Autodesk Inventor part; units mm, degrees
ref_plane "YZ Plane" through (0, 0, 0) normal (1, 0, 0) x (0, 1, 0)
ref_plane "XZ Plane" through (0, 0, 0) normal (0, 1, 0) x (-1, 0, 0)
ref_plane "XY Plane" through (0, 0, 0) normal (0, 0, 1) x (1, 0, 0)
sketch "Sketch1" plane through (0, 0, 0) normal (0, 0, 1) x (1, 0, 0)
  circle A0 centre (0, 0) radius 17.5
  dimension "d0" = 35
extrude "Extrusion1" add sketch "Sketch1" along normal blind 4.5
sketch "Sketch2" plane through (0, 0, 4.5) normal (0, 0, 1) x (1, 0, 0)
  circle A0 centre (0, 0) radius 17.5
  circle A1 centre (0, 0) radius 11
  dimension "d3" = 22
extrude "Extrusion2" add sketch "Sketch2" along normal blind 6.5 contours A1
sketch "Sketch3" plane through (0, 0, 11) normal (0, 0, 1) x (1, 0, 0)
  circle A0 centre (0, 0) radius 11
  circle A1 centre (0, 0) radius 6
  dimension "d6" = 12
extrude "Extrusion3" cut sketch "Sketch3" against normal through all contours A1
properties part number "culinder cap"
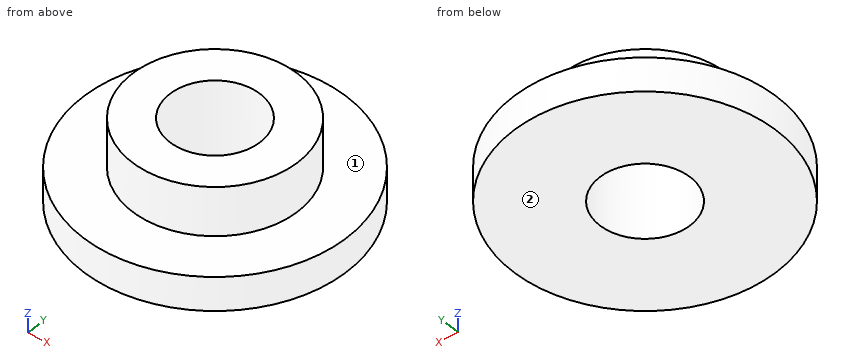
Geometry: final body of the model. Coordinates: model frame, mm. Face numbers are marked on the shaded views. A direction names the side the tool comes from. Round coordinates to 2 decimals unless told otherwise and drop trailing zeros. Loops run counter-clockwise (first coordinate to the right, second up) from the corner with the lowest first, then second, coordinate; pieces in that order, holes last. Notation, with made-up numbers: (-13.5, 14) -> (-8.5, 14) arc R22 ccw to (-8.5, 49) -> close; hole circle Ø10 at (78, 6). An arc over 180 degrees is marked (long way). Write each question's results on one line, items separated by ' | '.
Item 1: Pin query (flat end, axial travel): pin 1 Ø4 at (y, z) = (3.5, 6) entering from +X; pin 2 Ø1.5 at (x, y) = (-9, 10.5) entering from +Z; pin 3 Ø3 at (x, z) = (-7, 5) entering from -Y; pin 4 Ø7 at (x, y) = (0, 0) entering from -Z. Return the tip coordinate at first contact, or that it passes through.
Answers below:
pin 1: stops at x = 17.36 | pin 2: stops at z = 4.5 | pin 3: stops at y = -16.58 | pin 4: passes through
Item 2: Cut plane C-C on z = 5. Return the cut outline in (x, y).
Answers below:
outline: circle Ø22 at (0, 0); hole circle Ø12 at (0, 0)
Item 3: Set-up query: the marked faces 1 and 2. Return all of +Z, -Z, +X, -X, +Y, -Y with unobstructed straight access to the full face (end or side cutting, diameter ignored); none if empty.
Answers below:
face 1: +Z | face 2: -Z, +X, -X, +Y, -Y
Item 4: Line query: probe 1 along Y at (x, z) = (0, 9.25); probe 2 along Y at (x, z) = (0, 2.5); probe 3 along Z at (x, y) = (2, 13). Output: solid intervals per line, ascending. Write a range as [from, to].
Answers below:
probe 1: y = [-11, -6], [6, 11] | probe 2: y = [-17.5, -6], [6, 17.5] | probe 3: z = [0, 4.5]
Item 5: Cut plane D-D on y = 9. Return the cut outline in (x, z).
Answers below:
outline: (-15.01, 0) -> (15.01, 0) -> (15.01, 4.5) -> (6.32, 4.5) -> (6.32, 11) -> (-6.32, 11) -> (-6.32, 4.5) -> (-15.01, 4.5) -> close
Item 6: Cut plane A-A on y = 0. Return the cut outline in (x, z).
Answers below:
outline: (-17.5, 0) -> (-6, 0) -> (-6, 11) -> (-11, 11) -> (-11, 4.5) -> (-17.5, 4.5) -> close; (6, 0) -> (17.5, 0) -> (17.5, 4.5) -> (11, 4.5) -> (11, 11) -> (6, 11) -> close
